For this review, take the finished solid that the model builds, in its own axes (mm). Give positions to 0.01 mm unless a question says otherwise; leave off trailing zeros. Order: outer loops, then holes, each group sorted by start corner. A loop starts at its lowest first (then second) coordinate and runs counter-clockwise, first axis right, second up. Notation, with made-up numbers: (56.25, -19.5) - (103.25, -19.5) arc R13 cw to (103.25, -13.5) - close; hole circle Ø10 at (1.25, -3). An arc over 180 degrees is marked (long way). Use a Markdown table: item, result. Add a question column.
1) We need section B-B on y = -48. Write out the cut boundary in (x, z).
2) Wall thickness on L1, parallel to Y at x = -67.5, z = 2.4; L2, parallel to X at y = 35.5, z = 2; L3, parallel to Y at x = 28.1, z = 1.4: over which ranges is each line inside the solid? List them lowest first.
3) Clearance check with flat-ended pins moving along their axes: P1, Ø4, axis at x = 8.2, y = 8.3, coming from the +Z side; P2, Ø1, axis at y = 20, z = 0.5, coming from the -X side. State where each tip first meets the part, or that it passes through.
4) Mouldability with a two-part tool opening along Y and no side actions: class faces 1 (the face through (-67.8, 20.1, 1.5)), 2 (the face through (-155.13, -8.31, 1.48)), 3 (the face through (-31, -15, 0)), 4 (the face through (80.585, 0.651, 1.479)) as released by +Y, released by -Y, zero draft, split by the parting line, or undercut.
5) We need section A-A on z = 1. Give the number of separate pieces and of enclosed holes in the cut face, then the cut area to 3 significant figures.
```python
from build123d import *

# Parameters (mm, degrees)
SKETCH1_R           = 2
SKETCH1_R_2         = 2.5
SKETCH1_R_3         = 5.5
SKETCH1_R_4         = 1.75
SKETCH1_R_5         = 8.75
SKETCH1_R_6         = 16
BOSS_EXTRUDE1_DEPTH = 3


with BuildPart() as part:
    # Sketch1 → Boss-Extrude1 (new body)
    with BuildSketch(Plane.XY):
        with BuildLine():
            ThreePointArc((-113.560266524, 49.479735972), (-130.694234864, 42.395842918), (-136.329525131, 24.732380193))
            ThreePointArc((-136.329525131, 24.732380193), (-137.686520221, 16.356467092), (-143.370984404, 10.056925608))
            ThreePointArc((-143.370984404, 10.056925608), (-155.166532009, -8.626129333), (-147.542861296, -29.364285714))
            ThreePointArc((-147.542861296, -29.364285714), (-143.475887893, -32.124161339), (-138.735140925, -33.421275181))
            ThreePointArc((-138.735140925, -33.421275181), (-127.733357788, -40.106373668), (-125.965715234, -52.858048609))
            ThreePointArc((-125.965715234, -52.858048609), (-121.095745986, -74.463536322), (-99.899442585, -80.88462828))
            Line((-99.899442585, -80.88462828), (87.590338172, -36.326384859))
            ThreePointArc((87.590338172, -36.326384859), (89.625170423, -35.311295666), (91, -33.5))
            ThreePointArc((91, -33.5), (97.213976906, 3.543991621), (84.648444567, 38.941424032))
            ThreePointArc((84.648444567, 38.941424032), (82.945648013, 40.504860181), (80.721588123, 41.135261877))
            Line((80.721588123, 41.135261877), (-113.560266524, 49.479735972))
        make_face()
        with Locations((-138.3, -22.75)):
            Circle(SKETCH1_R, mode=Mode.SUBTRACT)
        with Locations((-68.3, -21.5)):
            Circle(SKETCH1_R_2, mode=Mode.SUBTRACT)
        with Locations((-138.3, -5.25)):
            Circle(SKETCH1_R, mode=Mode.SUBTRACT)
        with Locations((-74.1, 1.7)):
            Circle(SKETCH1_R_2, mode=Mode.SUBTRACT)
        with Locations((18.7, -8.7)):
            Circle(SKETCH1_R_2, mode=Mode.SUBTRACT)
        with Locations((76.2, -22)):
            Circle(SKETCH1_R_2, mode=Mode.SUBTRACT)
        with Locations((8.2, 8.3)):
            Circle(SKETCH1_R_2, mode=Mode.SUBTRACT)
        with Locations((36.382449965, 0)):
            Circle(SKETCH1_R_3, mode=Mode.SUBTRACT)
        with Locations((78.2, -0.1)):
            Circle(SKETCH1_R_2, mode=Mode.SUBTRACT)
        with Locations((28.1, 9)):
            Circle(SKETCH1_R_2, mode=Mode.SUBTRACT)
        with Locations((-112.981409671, 13.583075301)):
            Circle(SKETCH1_R_4, mode=Mode.SUBTRACT)
        with Locations((-128.421228626, 25.977105744)):
            Circle(SKETCH1_R_4, mode=Mode.SUBTRACT)
        with Locations((-65.3, 20)):
            Circle(SKETCH1_R_2, mode=Mode.SUBTRACT)
        with Locations((-114.504303927, 27.5)):
            Circle(SKETCH1_R_5, mode=Mode.SUBTRACT)
        with Locations((-100.587379227, 29.022894256)):
            Circle(SKETCH1_R_4, mode=Mode.SUBTRACT)
        with Locations((-116.027198182, 41.416924699)):
            Circle(SKETCH1_R_4, mode=Mode.SUBTRACT)
        with Locations((73.2, 22.3)):
            Circle(SKETCH1_R_2, mode=Mode.SUBTRACT)
        with Locations((-104.986214828, -59.480779371)):
            Circle(SKETCH1_R_6, mode=Mode.SUBTRACT)
    extrude(amount=BOSS_EXTRUDE1_DEPTH)


solid = part.part
```
Checked values:
| question | item | result |
|---|---|---|
| 1 | outline | (-125.27, 0) - (-116.13, 0) - (-116.13, 3) - (-125.27, 3) - close; (-93.84, 0) - (38.47, 0) - (38.47, 3) - (-93.84, 3) - close |
| 2 | L1 | -73.18 to -23.87, -19.13 to 18.81, 21.19 to 47.5 |
| 2 | L2 | -135 to -118.05, -110.96 to 86.84 |
| 2 | L3 | -50.46 to 6.5, 11.5 to 43.4 |
| 3 | P1 | through |
| 3 | P2 | x = -136.59 |
| 4 | face 1 | undercut |
| 4 | face 2 | split by the parting line |
| 4 | face 3 | zero draft |
| 4 | face 4 | undercut |
| 5 | separate pieces | 1 |
| 5 | enclosed holes | 18 |
| 5 | area | 23,300 mm² |
